Autodesk Fusion 360 part; units mm, degrees
sketch "Sketch1" plane through (0, 0, 0) normal (0, 0, 1) x (1, 0, 0)
  circle A0 centre (0, -26.6945) radius 3.075
  circle A1 centre (0, -26.6945) radius 5.075
  ellipse E0 centre (0, 15.9768) end of major axis (17.5, 15.9768) minor radius 15
  line L0 (-17.5, 15.9768) -> (17.5, 15.9768) construction
  line L1 (0, 0.9768) -> (0, 30.9768) construction
  line L2 (-4.9979, -27.5758) -> (-10.5694, 4.0217)
  line L3 (4.9979, -27.5758) -> (10.5694, 4.0217)
  line L4 (-2.8477, -22.4938) -> (-7.222, 2.3137)
  line L5 (7.2219, 2.3137) -> (2.8477, -22.4938)
  dimension "d1" = 6.15
  dimension "d2" = 2
  dimension "d3" = 35
  dimension "d4" = 30
  dimension "d5" = 10
  dimension "d6" = 10
  dimension "d7" = 3
  dimension "d8" = 3
extrude "Extrude1" add sketch "Sketch1" along normal blind 12 contours A1 | A1 E0 L3 L5 | A1 E0 L2 L4 | E0 makes body 1
sketch "Sketch2" plane through (0, 0, 12) normal (0, 0, 1) x (-1, 0, 0)
  circle A0 centre (0, 26.6945) radius 3.075
  ellipse E0 centre (0, -15.9768) end of major axis (-17.5, -15.9768) minor radius 15 (7.222, -2.3137) -> (-7.2219, -2.3137) ccw
  line L0 (-7.2219, -2.3137) -> (-2.8477, 22.4938)
  arc A1 (-2.8477, 22.4938) -> (2.8477, 22.4938) centre (0, 26.6945) ccw
  line L1 (2.8477, 22.4938) -> (7.222, -2.3137)
  arc A2 (4.9979, 27.5758) -> (-4.9979, 27.5758) centre (0, 26.6945) ccw
  line L2 (-4.9979, 27.5758) -> (-10.5694, -4.0217)
  ellipse E1 centre (0, -15.9768) end of major axis (-17.5, -15.9768) minor radius 15 (-10.5694, -4.0217) -> (10.5694, -4.0217) ccw
  line L3 (10.5694, -4.0217) -> (4.9979, 27.5758)
  circle A3 centre (0, 26.6945) radius 3.5
  dimension "d11" = 7
extrude "Extrude2" cut sketch "Sketch2" against normal blind 3 contours A3 bodies 1
extrude "Extrude3" add sketch "Sketch1" against normal blind 53 separate body contours E0 makes body 2
move_body "Move1" bodies 2 to x (1, 0, 0) y (0, 1, 0) z (0, 0, 1) at (0, 0, 65)
combine "Combine1" operation add target body 1 tool bodies 2
equation "d14 = -( 65 mm - 12 mm )"
Read the model definition and answer for the solid it produces. Units are mm, in the model's axes. A direction names the side the tool comes from. Give positions to 0.01 mm unless a question says otherwise; leave off trailing zeros. Order: outer loops, then holes, each group sorted by start corner. A loop starts at its lowest first (then second) coordinate and runs counter-clockwise, first axis right, second up.
(1) For faces 1 (the cylindrical face through (0.76, -23.28, 10.52)), 2 (the flat face through (-5.004, -10.264, 5.916)), 3 (the flat face through (0, 16, 65)), determine the directions among +Z, -Z, +X, -X, +Y, -Y from which every point of the face is accessible in a straight line to the end or side of a thin tool.
(2) For a pull along Y with two mould halves and no side action, classify faces 4 (the flat face through (5.065, -9.916, 5.916)), 5 (the flat face through (0, 7, 0)), 6 (the flat face through (-7.745, -11.998, 5.916)) as released by +Y, released by -Y, zero draft, split by the parting line, or undercut.
(3) Given pin 1 (2 mm diameter, centred on x = -2, z = 44.5, fed in from +Y); pin 2 (7.5 mm diameter, centred on x = 0.5, y = -26.5, fed in from +Z); pin 3 (3 mm diameter, centred on x = -7.5, z = 19, fed in from -Y), each flat-ended and moving along its own axis, determine where each tip first touches the part or whether it passes through.
(4) Straight lines are drawn through the part: L1, parallel to Y at x = -1, z = 7; L2, parallel to Z at x = 4.5, y = -27; L3, parallel to Y at x = 0.5, z = 13. For each, find the intervals that lie inside material, in ascending order.
(5) Find section A-A (y = -3.5). Give the vertices of the cut face in (x, z), plus the area to 3 significant figures.
(6) Find section B-B (x = 0). Give the number of separate pieces and of enclosed holes in the cut face, plus the area to 3 significant figures.
Result sheet:
1. face 1: +Z
1. face 2: +Z, -Z
1. face 3: +Z, +X, -X, +Y, -Y
2. face 4: undercut
2. face 5: zero draft
2. face 6: released by -Y
3. pin 1: stops at y = 30.95
3. pin 2: stops at z = 12
3. pin 3: stops at y = 1.89
4. L1: y = -31.67 to -29.6, -23.79 to -21.72, 1 to 30.95
4. L2: z = 0 to 12
4. L3: y = 0.98 to 30.97
5. outline: (-9.24, 0) - (-6.2, 0) - (-6.2, 12) - (-9.24, 12) - close; (6.2, 0) - (9.24, 0) - (9.24, 12) - (6.2, 12) - close
5. area: 73.1 mm2
6. separate pieces: 3
6. enclosed holes: 0
6. area: 2,000 mm2
